Verification items for the finished model (mm, model axes). A direction names the side the tool comes from. Give positions to 0.01 mm unless a question says otherwise; leave off trailing zeros. Order: outer loops, then holes, each group sorted by start corner. A loop starts at its lowest first (then second) coordinate and runs counter-clockwise, first axis right, second up.
from build123d import *

# Parameters (mm, degrees)
BOSS_EXTRUDE1_START = 196.208778
BOSS_EXTRUDE1_DEPTH = 10.16


with BuildPart() as part:
    # Sketch1 → Boss-Extrude1 (new body)
    with BuildSketch(Plane.XY.offset(BOSS_EXTRUDE1_START)):
        Polygon((-0.102720764, -24.506851212), (-500.385059294, -112.720125467), (-500.385059294, -412.720125467), (0, -412.720125467), (0, -335.42775434), (25, -335.42775434), (25, -254.110815755), (0, -254.110815755), (0, -172.79387717), (25, -172.79387717), (25, -91.476938585), (0, -91.476938585), align=None)
    extrude(amount=BOSS_EXTRUDE1_DEPTH)


solid = part.part
(1) Set-up check for faces 5 (the flat face through (0, -375, 201)), 6 (the flat face through (0, -214, 201)), 7 (the flat face through (13, -91.477, 201)): record each of +Z, -Z, +X, -X, +Y, -Y from which the full face is reachable in a straight line by a thin tool's end or side.
Solved:
face 5: +Z, -Z, +X, -Y
face 6: +Z, -Z, +X
face 7: +Z, -Z, +X, +Y
(2) Release check for a two-part mould opening along Y. For faces 1 (the flat face through (12, -172.794, 201)), 2 (the flat face through (-246.742, -67.996, 201.218)), 3 (the flat face through (-241, -259, 206.369)), 4 (the flat face through (13, -254.111, 201)) record: pulls with the +Y half, pulls with the -Y half, needs draft (parallel to the pull), parting line crosses it, or undercut.
Solved:
face 1: undercut
face 2: pulls with the +Y half
face 3: needs draft
face 4: undercut
(3) Section check A-A, the plane z = 200.75. Enter the section's corners in (x, y), then the cut area to 3 significant figures.
Solved:
outline: (-500.39, -412.72) - (0, -412.72) - (0, -335.43) - (25, -335.43) - (25, -254.11) - (0, -254.11) - (0, -172.79) - (25, -172.79) - (25, -91.48) - (0, -91.48) - (-0.1, -24.51) - (-500.39, -112.72) - close
area: 176,000 mm2
(4) Go/stop test with flat-tipped pins: pin 1 (4 mm diameter, centred on y = -361.5, z = 205, fed in from +X); pin 2 (3 mm diameter, centred on x = 10.5, z = 200.5, fed in from -Y). Record where each tip stops, or that it passes through.
Solved:
pin 1: stops at x = 0
pin 2: stops at y = -335.43
(5) Section check C-C, the plane x = -66.5. Enter the section's corners in (y, z).
Solved:
outline: (-412.72, 196.21) - (-36.21, 196.21) - (-36.21, 206.37) - (-412.72, 206.37) - close
(6) Scan lines: line 1 (X direction, y = -385, z = 198.25); line 2 (Y direction, x = -427, z = 199.25); line 3 (Y direction, x = -76, z = 201.25). Record each from-to range of solid material in increasing order.
Solved:
line 1: x = -500.39 to 0
line 2: y = -412.72 to -99.78
line 3: y = -412.72 to -37.89
(7) Section check B-B, the plane y = -180. Enter the section's corners in (x, z).
Solved:
outline: (-500.39, 196.21) - (0, 196.21) - (0, 206.37) - (-500.39, 206.37) - close
